Input: part model. Units: mm. Frame: model coordinates. A direction names the side the tool comes from. Coordinates: 2 decimals unless noted, no trailing zeros. Write each loop counter-clockwise with the first axis right and the second up, starting at its lowest first coordinate (ties: lowest second). Pieces come first, ordered by that corner, then holes. Notation, with made-up numbers: (73.5, 54.25) -> (119.5, 54.25) arc R28 cw to (119.5, 74.25) -> close; hole circle Ø1 at (59, 36.5). An arc over 180 degrees is marked (long way). Use one line per item in the form item = value. Start each with the question number.
(1) Cut plane A-A on z = -6. Return the cut outline in (x, y).
(2) Ray query, line 1 along X through (y, z) = (-32.5, -33.5); line 2 along Z through (x, y) = (10, -18); line 3 along Z through (x, y) = (15, -27). Return the intervals inside material, ascending.
(3) Cut plane B-B on y = -35.5. Return the cut outline in (x, z).
(4) Cut plane C-C on y = -11. Return the cut outline in (x, z), plus the area to 3 significant figures.
(5) Set-up query: faces 1 (the face through (18.33, -28.72, -32.17)), 2 (the face through (8.627, -1.578, -17.291)). Return all of +Z, -Z, +X, -X, +Y, -Y with unobstructed straight access to the full face (end or side cutting, diameter ignored); none if empty.
(6) First-contact query: pin 1 (4 mm diameter, centred on x = 15.19, z = 40.22, fed in from +Y); pin 2 (5.5 mm diameter, centred on x = 15.19, z = -33.48, fed in from -Y). Flat tips, straight axial feed; report the tip coordinate or a pass-through.
(7) Pull-direction query (X, two-part tool) for faces 3 (the face through (8.947, -21.858, 23.89)), 4 (the face through (-2.14, -20.28, 47.97)), 5 (the face through (15, 0, 3)); classes: released by +X, released by -X, zero draft, split by the parting line, or undercut.
(8) Cut plane D-D on x = 10. State how many separate pieces and enclosed holes the cut face has, plus the area to 3 significant figures.
```python
from build123d import *

# Parameters (mm, degrees)
SKETCH1_W             = 36.38
SKETCH1_H             = 91
BOSS_EXTRUDE1_DEPTH   = 40
FILLET1_R             = 3
CUT_EXTRUDE1_REACH    = 73.432
M8_TAPPED_HOLE1_D     = 6.8
M8_TAPPED_HOLE1_DEPTH = 22.25
M8_TAPPED_HOLE1_TIP   = 2.042926105


with BuildPart() as part:
    # Sketch1 → Boss-Extrude1 (new body)
    with BuildSketch(Plane(origin=(0, 0, 0), x_dir=(1, 0, 0), z_dir=(0, 1, 0))):
        with Locations((15.19, -3.37)):
            Rectangle(SKETCH1_W, SKETCH1_H)
    extrude(amount=-BOSS_EXTRUDE1_DEPTH)

    # Fillet1
    fillet1_edges = [part.edges().sort_by_distance(p)[0] for p in [
        (33.38, -20, 48.87),
        (-3, -20, 48.87),
        (-3, -20, -42.13),
        (33.38, -20, -42.13),
    ]]
    fillet(fillet1_edges, radius=FILLET1_R)

    # Sketch2 → Cut-Extrude1 (cut, up to next)
    with BuildSketch(Plane(origin=(0, 0, 0), x_dir=(1, 0, 0), z_dir=(0, 1, 0)), mode=Mode.PRIVATE) as cut_extrude1_sk1:
        with BuildLine():
            Line((28.43, 24.18), (4.88, 24.18))
            ThreePointArc((4.88, 24.18), (2.723324317, 23.286675683), (1.83, 21.13))
            Line((1.83, 21.13), (1.83, -27.87))
            ThreePointArc((1.83, -27.87), (2.723324317, -30.026675683), (4.88, -30.92))
            Line((4.88, -30.92), (28.43, -30.92))
            Line((28.43, -30.92), (28.43, -27.37))
            ThreePointArc((28.43, -27.37), (27.976015511, -26.273984489), (26.88, -25.82))
            Line((26.88, -25.82), (12.88, -25.82))
            ThreePointArc((12.88, -25.82), (8.672714652, -24.077285348), (6.93, -19.87))
            Line((6.93, -19.87), (6.93, 13.13))
            ThreePointArc((6.93, 13.13), (8.672714652, 17.337285348), (12.88, 19.08))
            Line((12.88, 19.08), (26.88, 19.08))
            ThreePointArc((26.88, 19.08), (27.976015511, 19.533984489), (28.43, 20.63))
            Line((28.43, 20.63), (28.43, 24.18))
        make_face()
    cut_extrude1_tool1 = extrude(cut_extrude1_sk1.sketch, amount=-CUT_EXTRUDE1_REACH, mode=Mode.PRIVATE) & part.part
    add(cut_extrude1_tool1.solids().sort_by_distance((6.318153, 0, 3.37))[0], mode=Mode.SUBTRACT)

    # Cut-Sweep1: sweep along a path in Sketch4
    with BuildLine(Plane(origin=(0, 0, 0), x_dir=(1, 0, 0), z_dir=(0, 1, 0))) as cut_sweep1_path:
        Line((28.43, 20.63), (28.43, 24.18))
        Line((28.43, 24.18), (4.88, 24.18))
        ThreePointArc((4.88, 24.18), (2.723324317, 23.286675683), (1.83, 21.13))
        Line((1.83, 21.13), (1.83, -27.87))
        ThreePointArc((1.83, -27.87), (2.723324317, -30.026675683), (4.88, -30.92))
        Line((4.88, -30.92), (28.43, -30.92))
        Line((28.43, -30.92), (28.43, -27.37))
        ThreePointArc((28.43, -27.37), (27.976015511, -26.273984489), (26.88, -25.82))
        Line((26.88, -25.82), (12.88, -25.82))
        ThreePointArc((12.88, -25.82), (8.672714652, -24.077285348), (6.93, -19.87))
        Line((6.93, -19.87), (6.93, 13.13))
        ThreePointArc((6.93, 13.13), (8.672714652, 17.337285348), (12.88, 19.08))
        Line((12.88, 19.08), (26.88, 19.08))
        ThreePointArc((26.88, 19.08), (27.976015511, 19.533984489), (28.43, 20.63))
    # Sketch3 → Cut-Sweep1 (sweep, cut)
    with BuildSketch(Plane.XY):
        Polygon((1.83, -3.2), (1.187653611, -40), (1.83, -40), align=None)
    sweep(path=cut_sweep1_path.line, transition=Transition.RIGHT, mode=Mode.SUBTRACT)

    # M8 Tapped Hole1
    with Locations(Plane(origin=(0, -40, 0), x_dir=(-1, 0, 0), z_dir=(0, -1, 0))):
        with Locations((-15.19, 33.476173195), (-15.19, -40.216173195)):
            Hole(M8_TAPPED_HOLE1_D / 2, depth=M8_TAPPED_HOLE1_DEPTH)
            with Locations((0, 0, -(M8_TAPPED_HOLE1_DEPTH + M8_TAPPED_HOLE1_TIP / 2))):  # 118° drill point
                Cone(0, M8_TAPPED_HOLE1_D / 2, M8_TAPPED_HOLE1_TIP, mode=Mode.SUBTRACT)


solid = part.part
```
Values:
q1.outline = (-3, -40) -> (1.19, -40) -> (1.83, -3.2) -> (1.83, 0) -> (-3, 0) -> close; (6.93, -3.2) -> (7.57, -40) -> (33.38, -40) -> (33.38, 0) -> (6.93, 0) -> close
q2.line_1 = -3 to 11.79, 18.59 to 33.38
q2.line_2 = -42.13 to -24.44, -18.04 to 24.78, 31.18 to 48.87
q2.line_3 = -42.13 to -36.87, -30.08 to -24.6, -18.66 to 25.4, 31.34 to 36.82, 43.61 to 48.87
q3.outline = (-3, -39.13) arc R3 ccw to (0, -42.13) -> (30.38, -42.13) arc R3 ccw to (33.38, -39.13) -> (33.38, 45.87) arc R3 ccw to (30.38, 48.87) -> (0, 48.87) arc R3 ccw to (-3, 45.87) -> close; hole (1.27, -21.13) arc R3.61 ccw to (4.88, -24.74) -> (28.99, -24.74) -> (28.99, -20.63) arc R2.11 ccw to (26.88, -18.52) -> (12.88, -18.52) arc R5.39 cw to (7.49, -13.13) -> (7.49, 19.87) arc R5.39 cw to (12.88, 25.26) -> (26.88, 25.26) arc R2.11 ccw to (28.99, 27.37) -> (28.99, 31.48) -> (4.88, 31.48) arc R3.61 ccw to (1.27, 27.87) -> close; hole circle Ø6.8 at (15.19, -33.48); hole circle Ø6.8 at (15.19, 40.22)
q4.outline = (-3, -39.13) arc R3 ccw to (0, -42.13) -> (30.38, -42.13) arc R3 ccw to (33.38, -39.13) -> (33.38, 45.87) arc R3 ccw to (30.38, 48.87) -> (0, 48.87) arc R3 ccw to (-3, 45.87) -> close; hole (1.69, -21.13) arc R3.19 ccw to (4.88, -24.32) -> (28.57, -24.32) -> (28.57, -20.63) arc R1.69 ccw to (26.88, -18.94) -> (12.88, -18.94) arc R5.81 cw to (7.07, -13.13) -> (7.07, 19.87) arc R5.81 cw to (12.88, 25.68) -> (26.88, 25.68) arc R1.69 ccw to (28.57, 27.37) -> (28.57, 31.06) -> (4.88, 31.06) arc R3.19 ccw to (1.69, 27.87) -> close
q4.area = 2,770 mm2
q5.face_1 = -Y
q5.face_2 = +Y, -Y
q6.pin_1 = 0
q6.pin_2 = -17.36
q7.face_3 = undercut
q7.face_4 = released by -X
q7.face_5 = zero draft
q8.separate_pieces = 3
q8.enclosed_holes = 0
q8.area = 3,120 mm2
